Can you work these out from the model? Positions are in its coordinate system, mm. A direction names the side the tool comes from. Coordinates: 2 decimals unless noted, no trailing zeros. Order: outer loops, then holes, each group sorted by start corner. A loop starts at its lowest first (then second) coordinate and runs counter-clockwise, first axis right, second up. Notation, with made-up numbers: (51.5, 46) - (71.5, 46) arc R8 ccw to (71.5, 56) - close; hole circle Ø1 at (86, -11). An arc over 180 degrees is marked (long way). Use a Markdown table: item, result. Add a question column.
(1) I want a section at C-C (z = 1.15). State how many separate pieces and enclosed holes the cut face has, and give its area (3 significant figures).
(2) If I drill on L1, parallel to Y at x = -70.5, z = 1.9; L2, parallel to X at y = 20.5, z = 2.85 (3 decimals); L3, parallel to Y at x = -6, z = 2.05, over which ranges is the centre line in solid material (lowest first)? Write a range as [from, to].
(3) On a 3-axis mill with a long thin cutter (end or side, diameter ignored), from which of +Z, -Z, +X, -X, +Y, -Y can I reach the whole of each face in a straight line? I mean faces 1 (the cylindrical face through (12.16, 17.35, 1.52)), 2 (the flat face through (71, -15.75, 1)), 3 (the cylindrical face through (-95.232, 52.824, 1.521)). Say none if no direction works.
(4) I want a section at A-A (x = 19). List the corners of the cut face in (y, z) for me, and give its area (3 significant figures).
(5) I want a section at B-B (x = -80). List the corners of the cut face in (y, z) for me.
(6) For pin 1 Ø4 at (x, y) = (45.415, 59.25) entering from +Z; pin 2 Ø0.9 at (x, z) = (-89, 1.5) entering from -Y, each with a flat end and sliding along its axis, tell me the tip position at first contact or that it passes through.
(7) We'd pull the mould along X, two halves only. Please class faces 4 (the cylindrical face through (50.586, -21.831, 1.479)), 5 (the flat face through (-9, 12.25, 1)), 6 (the flat face through (-89, -15.75, 1)), 7 (the cylindrical face through (-83.438, 55.676, 1.521)): pulls with the +X half, pulls with the -X half, needs draft (parallel to the pull), parting line crosses it, or undercut.
Autodesk Inventor part; units mm, degrees
ref_plane "YZ Plane" through (0, 0, 0) normal (1, 0, 0) x (0, 1, 0)
ref_plane "XZ Plane" through (0, 0, 0) normal (0, 1, 0) x (-1, 0, 0)
ref_plane "XY Plane" through (0, 0, 0) normal (0, 0, 1) x (1, 0, 0)
sketch "スケッチ1" plane through (0, 0, 0) normal (0, 0, 1) x (1, 0, 0)
  line L0 (-96.735, 64.25) -> (78.265, 64.25)
  line L1 (78.265, 64.25) -> (78.265, -25.75)
  line L2 (78.265, -25.75) -> (-96.735, -25.75)
  line L3 (-96.735, -25.75) -> (-96.735, 64.25)
  line L4 (-96.735, 64.25) -> (78.265, -25.75) construction
  line L5 (78.265, 64.25) -> (-96.735, -25.75) construction
  line L6 (-96.735, 19.25) -> (78.265, 19.25) construction
  line L7 (-96.735, 0) -> (78.265, 0) construction
  line L8 (-80, 4) -> (-80, -4) construction
  circle A0 centre (-80, -4) radius 1.6
  line L9 (0, 64.25) -> (0, -25.75) construction
  line L10 (19, -4) -> (19, 4) construction
  circle A1 centre (19, -4) radius 1.6
  circle A2 centre (-80, 4) radius 1.6
  circle A3 centre (19, 4) radius 1.6
  line L11 (16, 12.5) -> (22, 12.5) construction
  line L12 (22, 12.5) -> (22, -12.5) construction
  line L13 (22, -12.5) -> (16, -12.5) construction
  line L14 (16, -12.5) -> (16, 12.5) construction
  line L15 (16, 12.5) -> (22, -12.5) construction
  line L16 (22, 12.5) -> (16, -12.5) construction
  line L17 (-83, 12.5) -> (-77, 12.5) construction
  line L18 (-77, 12.5) -> (-77, -12.5) construction
  line L19 (-77, -12.5) -> (-83, -12.5) construction
  line L20 (-83, -12.5) -> (-83, 12.5) construction
  line L21 (-83, 12.5) -> (-77, -12.5) construction
  line L22 (-77, 12.5) -> (-83, -12.5) construction
  line L23 (-67, 49.25) -> (6, 49.25) construction
  line L24 (6, 49.25) -> (6, -10.75) construction
  line L25 (6, -10.75) -> (-67, -10.75) construction
  line L26 (-67, -10.75) -> (-67, 49.25) construction
  line L27 (-67, 49.25) -> (6, -10.75) construction
  line L28 (6, 49.25) -> (-67, -10.75) construction
  line L29 (-83, -4.5) -> (-83, 20.5) construction
  line L30 (-83, 20.5) -> (-77, 20.5) construction
  line L31 (-77, 20.5) -> (-77, -4.5) construction
  line L32 (-77, -4.5) -> (-83, -4.5) construction
  circle A4 centre (-80, 12) radius 1.6
  circle A5 centre (-80, 4) radius 1.6
  line L33 (16, 20.5) -> (22, 20.5) construction
  line L34 (16, -4.5) -> (16, 20.5) construction
  line L35 (22, -4.5) -> (16, -4.5) construction
  line L36 (22, 20.5) -> (22, -4.5) construction
  circle A6 centre (19, 4) radius 1.6
  circle A7 centre (19, 12) radius 1.6
  line L37 (-83, 3.5) -> (-83, 28.5) construction
  line L38 (-83, 28.5) -> (-77, 28.5) construction
  line L39 (-77, 28.5) -> (-77, 3.5) construction
  line L40 (-77, 3.5) -> (-83, 3.5) construction
  circle A8 centre (-80, 20) radius 1.6
  circle A9 centre (-80, 12) radius 1.6
  line L41 (16, 28.5) -> (22, 28.5) construction
  line L42 (16, 3.5) -> (16, 28.5) construction
  line L43 (22, 3.5) -> (16, 3.5) construction
  line L44 (22, 28.5) -> (22, 3.5) construction
  circle A10 centre (19, 12) radius 1.6
  circle A11 centre (19, 20) radius 1.6
  circle A12 centre (-80, -12) radius 1.6
  line L45 (-77, -20.5) -> (-83, -20.5) construction
  line L46 (-83, -20.5) -> (-83, 4.5) construction
  line L47 (-77, 4.5) -> (-77, -20.5) construction
  line L48 (16, -20.5) -> (16, 4.5) construction
  circle A13 centre (19, -12) radius 1.6
  line L49 (22, -20.5) -> (16, -20.5) construction
  line L50 (22, 4.5) -> (22, -20.5) construction
  line L51 (45.415, -24.7) -> (77.215, -24.7) construction
  line L52 (77.215, -16.8) -> (45.415, -16.8) construction
  line L53 (45.415, -16.8) -> (45.415, -24.7) construction
  line L54 (45.415, -24.7) -> (77.215, -16.8) construction
  line L55 (77.215, -24.7) -> (45.415, -16.8) construction
  line L56 (77.215, -20.75) -> (45.415, -20.75) construction
  line L57 (61.315, -24.7) -> (61.315, -16.8) construction
  circle A14 centre (45.415, -20.75) radius 1.6
  circle A15 centre (51.765, -20.75) radius 1.6
  line L58 (73.615, -19.1623) -> (73.615, -22.3377) construction
  line L59 (73.615, -22.3377) -> (70.865, -23.9254) construction
  line L60 (70.865, -23.9254) -> (68.115, -22.3377) construction
  line L61 (68.115, -22.3377) -> (68.115, -19.1623) construction
  line L62 (68.115, -19.1623) -> (70.865, -17.5746) construction
  line L63 (70.865, -17.5746) -> (73.615, -19.1623) construction
  line L64 (-9.235, 64.25) -> (-9.235, -25.75) construction
  circle A16 centre (45.415, 59.25) radius 1.6
  circle A17 centre (51.765, 59.25) radius 1.6
  line L65 (73.615, 57.6623) -> (73.615, 60.8377) construction
  line L66 (73.615, 60.8377) -> (70.865, 62.4254) construction
  line L67 (70.865, 62.4254) -> (68.115, 60.8377) construction
  line L68 (68.115, 60.8377) -> (68.115, 57.6623) construction
  line L69 (68.115, 57.6623) -> (70.865, 56.0746) construction
  line L70 (70.865, 56.0746) -> (73.615, 57.6623) construction
  circle A18 centre (-63.885, -20.75) radius 1.6
  circle A19 centre (-70.235, -20.75) radius 1.6
  line L71 (-92.085, -19.1623) -> (-92.085, -22.3377) construction
  line L72 (-92.085, -22.3377) -> (-89.335, -23.9254) construction
  line L73 (-89.335, -23.9254) -> (-86.585, -22.3377) construction
  line L74 (-86.585, -22.3377) -> (-86.585, -19.1623) construction
  line L75 (-86.585, -19.1623) -> (-89.335, -17.5746) construction
  line L76 (-89.335, -17.5746) -> (-92.085, -19.1623) construction
  circle A20 centre (-63.885, 59.25) radius 1.6
  circle A21 centre (-70.235, 59.25) radius 1.6
  line L77 (-86.585, 57.6623) -> (-89.335, 56.0746) construction
  line L78 (-86.585, 60.8377) -> (-86.585, 57.6623) construction
  line L79 (-89.335, 62.4254) -> (-86.585, 60.8377) construction
  line L80 (-92.085, 60.8377) -> (-89.335, 62.4254) construction
  line L81 (-92.085, 57.6623) -> (-92.085, 60.8377) construction
  line L82 (-89.335, 56.0746) -> (-92.085, 57.6623) construction
  line L83 (-34.235, 49.25) -> (15.765, 49.25) construction
  line L84 (15.765, 49.25) -> (15.765, 9.25) construction
  line L85 (15.765, 9.25) -> (-34.235, 9.25) construction
  line L86 (-34.235, 9.25) -> (-34.235, 49.25) construction
  line L87 (-34.235, 49.25) -> (15.765, 9.25) construction
  line L88 (15.765, 49.25) -> (-34.235, 9.25) construction
  line L89 (-31.235, 46.25) -> (12.765, 46.25) construction
  line L90 (12.765, 46.25) -> (12.765, 12.25) construction
  line L91 (12.765, 12.25) -> (-31.235, 12.25) construction
  line L92 (-31.235, 12.25) -> (-31.235, 46.25) construction
  line L93 (-31.235, 46.25) -> (12.765, 12.25) construction
  line L94 (12.765, 46.25) -> (-31.235, 12.25) construction
  circle A22 centre (-31.235, 12.25) radius 1.6
  circle A23 centre (-31.235, 46.25) radius 1.6
  circle A24 centre (12.765, 46.25) radius 1.6
  circle A25 centre (12.765, 12.25) radius 1.6
  line L95 (-62, -21.85) -> (-61.735, -21.85)
  line L96 (77.215, -16.8) -> (77.215, -24.7) construction
  line L97 (63.465, -25.75) -> (63.465, -15.75)
  line L98 (63.465, -15.75) -> (78.265, -15.75)
  line L99 (70.865, -23.9254) -> (70.865, -17.5746) construction
  line L100 (63.465, 64.25) -> (63.465, 54.25)
  line L101 (63.465, 54.25) -> (78.265, 54.25)
  line L102 (-81.935, -25.75) -> (-81.935, -15.75)
  line L103 (-81.935, -15.75) -> (-96.735, -15.75)
  line L104 (-81.935, 54.25) -> (-96.735, 54.25)
  line L105 (-81.935, 64.25) -> (-81.935, 54.25)
  line L106 (-9.235, 49.25) -> (-9.235, 9.25) construction
  circle A26 centre (35.765, 31.5525) radius 1.5
  circle A27 centre (35.765, 41.5525) radius 1.5
  line L107 (35.765, 31.5525) -> (35.765, 41.5525) construction
  line L108 (-34.235, 29.25) -> (15.765, 29.25) construction
  circle A28 centre (35.765, 26.9475) radius 1.5
  circle A29 centre (35.765, 16.9475) radius 1.5
  circle A30 centre (-54.235, 31.5525) radius 1.5
  circle A31 centre (-54.235, 41.5525) radius 1.5
  circle A32 centre (-54.235, 26.9475) radius 1.5
  circle A33 centre (-54.235, 16.9475) radius 1.5
  circle A34 centre (-16.735, -10.75) radius 1.5
  circle A35 centre (-1.735, -10.75) radius 1.5
  line L109 (-1.735, -10.75) -> (-16.735, -10.75) construction
  arc A36 (-27.235, 12.25) -> (-31.235, 16.25) centre (-31.235, 12.25) ccw
  line L110 (-31.235, 16.25) -> (-31.235, 42.25)
  line L111 (-27.235, 12.25) -> (8.765, 12.25)
  arc A37 (12.765, 16.25) -> (8.765, 12.25) centre (12.765, 12.25) ccw
  line L112 (12.765, 16.25) -> (12.765, 42.25)
  arc A38 (-31.235, 42.25) -> (-27.235, 46.25) centre (-31.235, 46.25) ccw
  line L113 (-27.235, 46.25) -> (8.765, 46.25)
  arc A39 (8.765, 46.25) -> (12.765, 42.25) centre (12.765, 46.25) ccw
  point P0 (0, 0)
  point P1 (-9.235, 19.25)
  point P2 (-80, 0)
  point P3 (19, 0)
  point P4 (-30.5, 19.25)
  point P5 (61.315, -20.75)
  point P6 (70.865, -20.75)
  point P7 (-9.235, 29.25)
  point P8 (-9.235, 29.25)
  point P9 (-9.235, 29.25)
  point P10 (35.765, 36.5525)
  point P11 (-9.235, -10.75)
  dimension "d0" = 175
  dimension "d1" = 90
  dimension "d2" = 25.75
  dimension "d3" = 3.2
  dimension "d4" = 8
  dimension "d5" = 8
  dimension "d6" = 3.2
  dimension "d16" = 78.265
  dimension "d17" = 6
  dimension "d18" = 25
  dimension "d19" = 22
  dimension "d20" = 6
  dimension "d21" = 25
  dimension "d22" = 105
  dimension "d23" = 15
  dimension "d24" = 15
  dimension "d25" = 10
  dimension "d26" = 10
  dimension "d57" = 8
  dimension "d64" = 8
  dimension "d69" = 31.8
  dimension "d70" = 7.9
  dimension "d72" = 3.2
  dimension "d75" = 5.5
  dimension "d79" = 50
  dimension "d80" = 40
  dimension "d81" = 44
  dimension "d82" = 34
  dimension "d83" = 3.2
  dimension "d88" = 10
  dimension "d89" = 87.5
  dimension "d102" = 19.1
  dimension "d103" = 5
  dimension "d104" = 1.05
  dimension "d105" = 7.4
  dimension "d106" = 1.05
  dimension "d107" = 3
  dimension "d109" = 20
  dimension "d110" = 10
  dimension "d111" = 7.3025
  dimension "d112" = 42.765
  dimension "d113" = 10
  dimension "d114" = 15
  dimension "d115" = 20
  dimension "d116" = 4
extrude "押し出し1" add sketch "スケッチ1" along normal blind 3 contours L0 L100 L101 L1 L98 L97 L2 L102 L103 L3 L104 L105 | A4 | A7 | A8 | A11 | A12 | A13
fillet "フィレット1" radius 5 20 edges at (-81.935, -25.75, 1.5) (-81.935, -15.75, 1.5) (-96.735, -15.75, 1.5) (-96.735, 54.25, 1.5) (-81.935, 54.25, 1.5) (-81.935, 64.25, 1.5) (63.465, 64.25, 1.5) (63.465, 54.25, 1.5) (78.265, 54.25, 1.5) (78.265, -15.75, 1.5) (63.465, -25.75, 1.5) (63.465, -15.75, 1.5) (-27.235, 12.25, 1.5) (-31.235, 16.25, 1.5) (-31.235, 42.25, 1.5) (-27.235, 46.25, 1.5) (8.765, 46.25, 1.5) (12.765, 42.25, 1.5) (12.765, 16.25, 1.5) (8.765, 12.25, 1.5)
equation "\"d3\" = d6"
equation "\"d4\" = d5"
equation "\"d20\" = d17"
equation "\"d21\" = d18"
properties part number "Sole_frame" material "GFRP"
Answers follow:
| question | item | result |
|---|---|---|
| 1 | separate pieces | 1 |
| 1 | enclosed holes | 27 |
| 1 | area | 13,500 mm² |
| 2 | L1 | y = [-25.75, -22.33], [-19.17, 57.67], [60.83, 64.25] |
| 2 | L2 | x = [-96.735, -31.235], [12.765, 78.265] |
| 2 | L3 | y = [-25.75, 12.25], [46.25, 64.25] |
| 3 | face 1 | +Z, -Z |
| 3 | face 2 | +Z, -Z, +X, -Y |
| 3 | face 3 | +Z, -Z, -X, +Y |
| 4 | outline | (-25.75, 0) - (-5.6, 0) - (-5.6, 3) - (-25.75, 3) - close; (-2.4, 0) - (2.4, 0) - (2.4, 3) - (-2.4, 3) - close; (5.6, 0) - (64.25, 0) - (64.25, 3) - (5.6, 3) - close |
| 4 | area | 251 mm² |
| 5 | outline | (-24.7, 0) - (-5.6, 0) - (-5.6, 3) - (-24.7, 3) - close; (-2.4, 0) - (2.4, 0) - (2.4, 3) - (-2.4, 3) - close; (5.6, 0) - (63.2, 0) - (63.2, 3) - (5.6, 3) - close |
| 6 | pin 1 | stops at z = 3 |
| 6 | pin 2 | stops at y = -15.75 |
| 7 | face 4 | undercut |
| 7 | face 5 | undercut |
| 7 | face 6 | needs draft |
| 7 | face 7 | pulls with the -X half |
